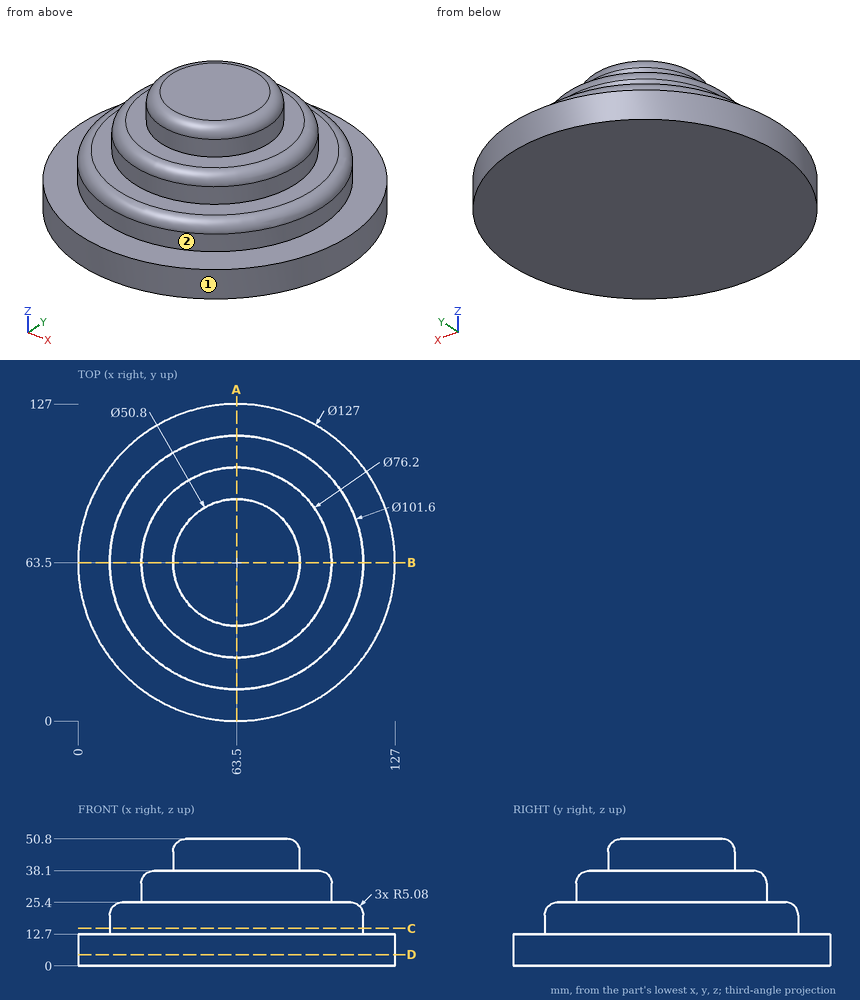
For this review, use the dimensioned drawing (mm, ordinates from the lowest corner) and the shaded views. A direction names the side the tool comes from. Give positions to 0.01 mm unless a question says otherwise; leave off trailing zeros. Write each loop counter-clockwise with the first axis right and the second up, starting at its lowest first coordinate (ties: lowest second). Pieces come first, ordered by that corner, then holes.
(1) To check wall thickness, follow L1, parallel to Z at x = 37.5, y = 77.5; L2, parallel to Z at x = 93, y = 110; L3, parallel to X at y = 17.5, z = 10 (3 decimals). State the ranges of each line that lie inside material, in increasing order.
(2) Consider section D-D, the plane z = 4.5. Give the boundary of the cut face in (x, y).
(3) Consider section C-C, the plane z = 15. Give the boundary of the cut face in (x, y).
(4) Tool access review of the marked faces 1 and 2: name each direction out of +Z, -Z, +X, -X, +Y, -Y from which nothing blocks a thin tool from reaching the whole face with its end or side.
(5) For P1, Ø8, axis at y = 77, z = 20.5, coming from the +X side; P2, Ø8, axis at y = 64, z = 25.5, coming from the -X side; P3, Ø3, axis at x = 74, y = 30, coming from the +Z side, all flat-tipped, find the tip position at first contact; note any pin that passes through.
(6) Consider section A-A, the plane x = 63.5. Give the boundary of the cut face in (y, z).
Returned:
1. L1: z = 0 to 38.1
1. L2: z = 0 to 12.7
1. L3: x = 19.725 to 107.275
2. outline: circle Ø127 at (63.5, 63.5)
3. outline: circle Ø101.6 at (63.5, 63.5)
4. face 1: +Z, -Z
4. face 2: +Z
5. P1: stops at x = 113.4
5. P2: stops at x = 12.84
5. P3: stops at z = 38.07
6. outline: (0, 0) - (127, 0) - (127, 12.7) - (114.3, 12.7) - (114.3, 20.32) arc R5.08 ccw to (109.22, 25.4) - (101.6, 25.4) - (101.6, 33.02) arc R5.08 ccw to (96.52, 38.1) - (88.9, 38.1) - (88.9, 45.72) arc R5.08 ccw to (83.82, 50.8) - (43.18, 50.8) arc R5.08 ccw to (38.1, 45.72) - (38.1, 38.1) - (30.48, 38.1) arc R5.08 ccw to (25.4, 33.02) - (25.4, 25.4) - (17.78, 25.4) arc R5.08 ccw to (12.7, 20.32) - (12.7, 12.7) - (0, 12.7) - close
